Geometry check sheet. Reference: the model listing, model coordinates, mm. A direction names the side the tool comes from. Round coordinates to 2 decimals unless told otherwise and drop trailing zeros. Write each loop counter-clockwise with the first axis right and the second up, starting at its lowest first coordinate (ties: lowest second). Pieces come first, ordered by that corner, then holes.
Item 1: Cross-section at A-A (x = 0). Enter the section's corners in (y, z).
Item 2: Access from +Z, -Z, +X, -X, +Y, -Y to the whole of each face (thin tool, end or side, straight path). Record for faces 1 (the face through (0, 0, 0)), 2 (the face through (-5.961, -26.846, 122.86)), 3 (the face through (-13.2, -24.3, 60)), 4 (the face through (-1.08, -4.88, 9.86)).
Item 3: Cross-section at D-D (z = 66.5). Enter the section's corners in (x, y), then the cut area to 3 significant figures.
Item 4: Scan lines: probe 1 along Z at (x, y) = (6, 20); probe 2 along Y at (x, z) = (0, 128.5); probe 3 along Y at (x, z) = (10, 69.5). Record each from-to range of solid material in increasing order.
Item 5: Cross-section at C-C (z = 115). Enter the section's corners in (x, y), then the cut area to 3 significant figures.
Item 6: Depth check by flat-ended pin: P1, Ø6, axis at x = 0, y = 0, coming from the -Z side; P2, Ø5, axis at x = 14, z = 56.5, coming from the -Y side; P3, Ø8, axis at x = 11, z = 115, coming from the -Y side; P4, Ø10, axis at y = 20.5, z = 86, coming from the +X side. Enter the tip coordinate at first touch or a pass-through.
Item 7: Draft check along X on faces 5 (the face through (29.97, 1.32, 50.14)), 6 (the face through (-1.08, -4.88, 122.86)), 7 (the face through (-13.2, -24.3, 40)). Enter one of: pulls with the +X half, pulls with the -X half, needs draft (parallel to the pull), parting line crosses it, or undercut.
from build123d import *

# Parameters (mm, degrees)
SKETCH1_R                = 5
BOSS_EXTRUDE1_DEPTH      = 20
SKETCH2_R                = 27.5
BOSS_EXTRUDE2_DEPTH      = 113
BOSS_EXTRUDE3_DEPTH      = 10
BOSS_EXTRUDE3_DEPTH_BACK = 10
SKETCH3_R                = 30
BOSS_EXTRUDE4_DEPTH      = 10
BOSS_EXTRUDE4_DEPTH_BACK = 10
SKETCH4_R                = 30
CUT_EXTRUDE1_START       = -20
SKETCH5_R                = 5
CUT_EXTRUDE1_DEPTH       = 20


with BuildPart() as part:
    # Sketch1 → Boss-Extrude1 (new body)
    with BuildSketch(Plane.XY):
        Circle(SKETCH1_R)
    extrude(amount=BOSS_EXTRUDE1_DEPTH)

    # Sketch2 → Boss-Extrude2 (add)
    with BuildSketch(Plane.XY.offset(20)):
        Circle(SKETCH2_R)
    extrude(amount=BOSS_EXTRUDE2_DEPTH)

    # Sketch3 → Boss-Extrude3 (add, two sides: drawn at the far end of the back side and taken through both)
    with BuildSketch(Plane(origin=(0, 0, 50), x_dir=(-1, 0, 0), z_dir=(0, 0, -1)).offset(-BOSS_EXTRUDE3_DEPTH_BACK)):
        Circle(SKETCH3_R)
    extrude(amount=BOSS_EXTRUDE3_DEPTH + BOSS_EXTRUDE3_DEPTH_BACK)

    # Sketch4 → Boss-Extrude4 (add, two sides: drawn at the far end of the back side and taken through both)
    with BuildSketch(Plane(origin=(0, 0, 103), x_dir=(-1, 0, 0), z_dir=(0, 0, -1)).offset(-BOSS_EXTRUDE4_DEPTH_BACK)):
        Circle(SKETCH4_R)
    extrude(amount=BOSS_EXTRUDE4_DEPTH + BOSS_EXTRUDE4_DEPTH_BACK)

    # Sketch5 → Cut-Extrude1 (cut)
    with BuildSketch(Plane.XY.offset(133).offset(CUT_EXTRUDE1_START)):
        Circle(SKETCH5_R)
    extrude(amount=CUT_EXTRUDE1_DEPTH, mode=Mode.SUBTRACT)


solid = part.part
Resolved:
1. outline: (-30, 40) - (-27.5, 40) - (-27.5, 20) - (-5, 20) - (-5, 0) - (5, 0) - (5, 20) - (27.5, 20) - (27.5, 40) - (30, 40) - (30, 60) - (27.5, 60) - (27.5, 93) - (30, 93) - (30, 113) - (27.5, 113) - (27.5, 133) - (5, 133) - (5, 113) - (-5, 113) - (-5, 133) - (-27.5, 133) - (-27.5, 113) - (-30, 113) - (-30, 93) - (-27.5, 93) - (-27.5, 60) - (-30, 60) - close
2. face 1: -Z, +X, -X, +Y, -Y
2. face 2: +Z
2. face 3: none
2. face 4: -Z
3. outline: circle Ø55 at (0, 0)
3. area: 2,380 mm2
4. probe 1: z = 20 to 133
4. probe 2: y = -27.5 to -5, 5 to 27.5
4. probe 3: y = -25.62 to 25.62
5. outline: circle Ø55 at (0, 0); hole circle Ø10 at (0, 0)
5. area: 2,300 mm2
6. P1: stops at z = 0
6. P2: stops at y = -27.71
6. P3: stops at y = -29.04
6. P4: stops at x = 22.72
7. face 5: parting line crosses it
7. face 6: undercut
7. face 7: needs draft
